from build123d import *


with BuildPart() as part:
    # Schizzo1 → Rivoluzione1 (revolve)
    with BuildSketch(Plane(origin=(0, 0, 0), x_dir=(0, 0, -1), z_dir=(1, 0, 0)), mode=Mode.PRIVATE) as rivoluzione1_sk:
        Polygon((24.193102917, 11.737734445), (24.193102917, -3.262265555), (25.77022715, -3.392816036), (25.77022715, 12.407183964), (-26.71449517, 72.783950382), (-28.291619402, 72.114500863), align=None)
        Polygon((-59.550109681, 145.754889139), (-28.291619402, 72.114500863), (-26.71449517, 72.783950382), (-57.688820987, 145.754889139), (-66.872170267, 180.027615233), (-70.49877626, 193.562293059), (-78.40877626, 193.562293059), (-78.40877626, 169.562293059), (-76.60877626, 169.562293059), (-76.60877626, 179.562293059), (-68.60877626, 179.562293059), align=None)
    revolve(rivoluzione1_sk.sketch.rotate(Axis((0, -3.392816036, -30.77022715), (0, 1, 0)), 180), axis=Axis((0, -3.392816036, -30.77022715), (0, 1, 0)))


solid = part.part
Verification items for the finished model (mm, model axes). A direction names the side the tool comes from. Give positions to 0.01 mm unless a question says otherwise; leave off trailing zeros. Write each loop counter-clockwise with the first axis right and the second up, starting at its lowest first coordinate (ties: lowest second). Pieces come first, ordered by that corner, then holes. Notation, with made-up numbers: (89, -6) - (115, -6) arc R20 ccw to (115, 17) - close; hole circle Ø3 at (-17.5, 35). An arc over 180 degrees is marked (long way). Answer as CSV lines item,"result". Start each with the question number.
1. Set-up check for faces 4 (the face through (106.583, 181.394, -7.102)), 5 (the face through (65.34, 174.63, 54.44)): record each of +Z, -Z, +X, -X, +Y, -Y from which the full face is reachable in a straight line by a thin tool's end or side.
2. Sectioned sample at A-A (y = 174). Record the boundary of the cut face in (x, z).
3. Thickness scan on line 1 (X direction, y = 170, z = -82); line 2 (Z direction, x = 31.5, y = 185); line 3 (Z direction, x = 21.5, y = 161.5). Record the ranges inside material, lowest first.
4. Sectioned sample at B-B (y = 34). Record the boundary of the cut face in (x, z).
5. Draft check along Z on faces 1 (the face through (72, 169.562, -111)), 2 (the face through (17.7, 29.6, -39.97)), 3 (the face through (-19.24, 83.872, -91.865)). Enter one of: pulls with the +Z half, pulls with the -Z half, needs draft (parallel to the pull), parting line crosses it, or undercut.
6. Depth check by flat-ended pin: pin 1 (6 mm diameter, centred on y = 97, z = -78, fed in from -X); pin 2 (2 mm diameter, centred on x = -83, z = -35.5, fed in from -Y); pin 3 (10 mm diameter, centred on y = 58, z = -43, fed in from +X) (3 decimals). Enter the tip coordinate at first touch or a pass-through.
Derived:
1,face 4,"+Y, -Y"
1,face 5,"-Y"
2,outline,"circle Ø218.36 at (0, -30.77); circle Ø195.78 at (0, -30.77); hole circle Ø214.76 at (0, -30.77); hole circle Ø192.05 at (0, -30.77)"
3,line 1,"-96.41 to -94.37, -82.15 to -79.95, 79.95 to 82.15, 94.37 to 96.41"
3,line 2,"-135.31 to -124.6, 63.06 to 73.77"
3,line 3,"-122.83 to -120.92, 59.38 to 61.29"
4,outline,"circle Ø51.86 at (0, -30.77); hole circle Ø47.54 at (0, -30.77)"
5,face 1,"needs draft"
5,face 2,"undercut"
5,face 3,"parting line crosses it"
6,pin 1,"x = -54.27"
6,pin 2,"y = 126.47"
6,pin 3,"x = 49.805"
